Check sheet for the modelled part. Datum: model origin and axes. Units: mm. Give positions to 0.01 mm unless a question says otherwise; leave off trailing zeros. Order: outer loops, then holes, each group sorted by start corner. A loop starts at its lowest first (then second) coordinate and runs counter-clockwise, first axis right, second up.
Item 1: Release check for a two-part mould opening along Z. For faces 1 (the flat face through (0, 0, 88.2)), 2 (the flat face through (0, 0, 0)) record: released by +Z, released by -Z, zero draft, split by the parting line, or undercut.
Item 2: Material ranges on line 1 along X through (y, z) = (-0.3, 36); line 2 along Y through (x, z) = (0.15, 36.5); line 3 along X through (y, z) = (-2.2, 75.5), recorded low to high.
Item 3: Sectioned sample at A-A on x = -0.7. Record the boundary of the cut face in (y, z), and give its area (3 significant figures).
Item 4: Sectioned sample at B-B on z = 45. Record the boundary of the cut face in (x, y), and give its area (3 significant figures).
Item 5: Sectioned sample at C-C on y = 1.4. Record the boundary of the cut face in (x, z).
from build123d import *

# Parameters (mm, degrees)
SKETCH_1_R             = 2.5
EXTRUDE_1_DEPTH        = 88.2
SKETCH_2_R             = 12.5
EXTRUDE_2_DEPTH        = 62
SKETCH_3_W             = 40
SKETCH_3_H             = 17.730441408
SKETCH_3_R             = 5
EXTRUDE_3_DEPTH        = 3
PATTERN_LINEAR_1_COUNT = 2
PATTERN_LINEAR_1_PITCH = 59
SKETCH_5_R             = 2.5
CUT_EXTRUDE_1_DEPTH    = 98.649833589


with BuildPart() as part:
    # 草图1 → 凸台-拉伸1 (new body)
    with BuildSketch(Plane.XY):
        Circle(SKETCH_1_R)
    extrude(amount=EXTRUDE_1_DEPTH)

    # 草图2 → 凸台-拉伸2 (add)
    with BuildSketch(Plane.XY.offset(73.2)):
        Circle(SKETCH_2_R)
    extrude(amount=-EXTRUDE_2_DEPTH)

    # 草图3 → 凸台-拉伸3 (add)
    with BuildSketch(Plane.XY.offset(73.2)):
        with Locations((20, 0)):
            Rectangle(SKETCH_3_W, SKETCH_3_H)
        with Locations((32.640039451, 0)):
            Circle(SKETCH_3_R, mode=Mode.SUBTRACT)
    extrude_3 = extrude(amount=-EXTRUDE_3_DEPTH)

    # 阵列(线性)1: 凸台-拉伸3 ×2
    with Locations(*[(0, 0, -i * PATTERN_LINEAR_1_PITCH) for i in range(1, PATTERN_LINEAR_1_COUNT)]):
        add(extrude_3)

    # 草图5 → 切除-拉伸1 (cut, through all)
    with BuildSketch(Plane.XY.offset(88.2)):
        with BuildLine():
            Line((8.812369821, 8.865220704), (40, 8.865220704))
            Line((40, 8.865220704), (40, -8.865220704))
            Line((40, -8.865220704), (8.812369821, -8.865220704))
            ThreePointArc((8.812369821, -8.865220704), (-12.5, 0), (8.812369821, 8.865220704))
        make_face()
        Circle(SKETCH_5_R, mode=Mode.SUBTRACT)
    extrude(amount=-CUT_EXTRUDE_1_DEPTH, mode=Mode.SUBTRACT)


solid = part.part
Report:
1. face 1: released by +Z
1. face 2: released by -Z
2. line 1: x = -2.48 to 2.48
2. line 2: y = -2.5 to 2.5
2. line 3: x = -1.19 to 1.19
3. outline: (-2.4, 0) - (2.4, 0) - (2.4, 88.2) - (-2.4, 88.2) - close
3. area: 423 mm2
4. outline: circle Ø5 at (0, 0)
4. area: 19.6 mm2
5. outline: (-2.07, 0) - (2.07, 0) - (2.07, 88.2) - (-2.07, 88.2) - close
